Could you check a few things on this drawing? It's one solid part, dimensions in mm from its lowest x, y, z. Give positions to 0.01 mm unless a question says otherwise; leave off trailing zeros. Loops run counter-clockwise (first coordinate to the right, second up) from the corner with the lowest first, then second, coordinate; pieces in that order, holes last. Notation, with made-up numbers: (43.5, 89) - (65.5, 89) arc R24 ccw to (65.5, 124) - close; hole circle Ø5 at (68, 59). An arc over 180 degrees is marked (long way). Return JSON: item names as keys, results as strings. Group by question number.
(1) I need wall thicknesses on probe 1 along Z at (x, y) = (202, 2); probe 2 along Z at (x, y) = (184, 1); probe 3 along X at (y, z) = (0.5, 58). Which ranges of each line are inside material? Lowest first, please. Write a range as [from, to].
(2) For P1, Ø1, axis at x = 84, z = 132.5, coming from the -Y side; P2, Ø3, axis at y = 3, z = 10, coming from the +X side; P3, Ø1, axis at x = 58.5, y = 2.5, coming from the -Z side; P4, Ø1.9, axis at x = 193, y = 4, coming from the +Z side, each with a flat end and sliding along its axis, tell me the tip position at first contact or that it passes through.
(3) If we section it at B-B (x = 72.5): Please give me the cut outline in (y, z), then the cut area to 3 significant figures.
(4) If we section it at A-A (z = 69): Please give me the cut outline in (x, y), then the cut area to 3 significant figures.
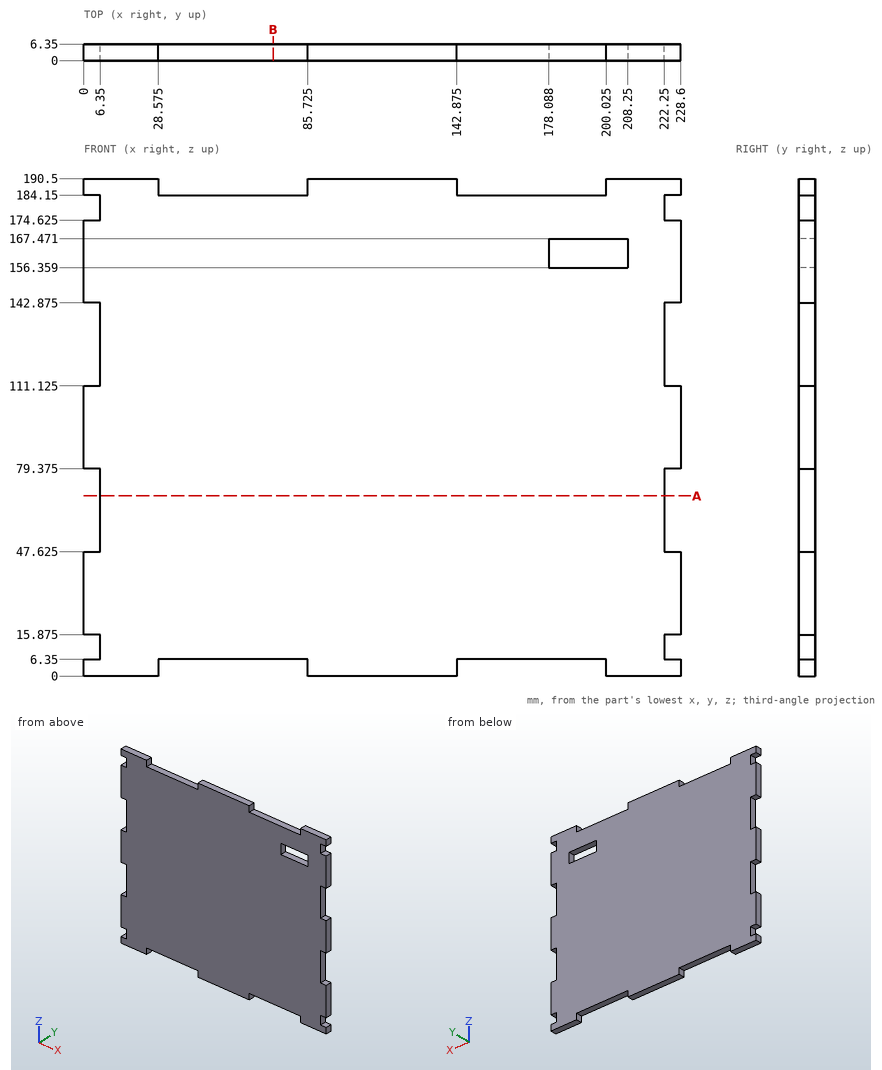
Values:
{
 "1": {"probe 1": "[0, 156.36], [167.47, 190.5]", "probe 2": "[6.35, 156.36], [167.47, 184.15]", "probe 3": "[6.35, 222.25]"},
 "2": {"P1": "y = 0", "P2": "x = 222.25", "P3": "z = 6.35", "P4": "z = 184.15"},
 "3": {"outline": "(0, 6.35) - (6.35, 6.35) - (6.35, 184.15) - (0, 184.15) - close", "area": "1,130 mm2"},
 "4": {"outline": "(6.35, 0) - (222.25, 0) - (222.25, 6.35) - (6.35, 6.35) - close", "area": "1,370 mm2"}
}
